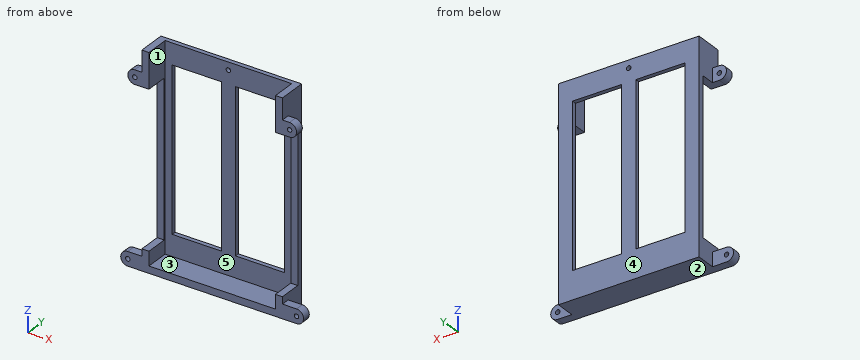
```python
from build123d import *

# Parameters (mm, degrees)
SKETCH_2_W          = 100
SKETCH_2_H          = 40
EXTRUDE_1_DEPTH     = 150
SKETCH_3_W          = 90
SKETCH_3_H          = 32
CUT_EXTRUDE_1_DEPTH = 145
SKETCH_4_W          = 30
SKETCH_4_H          = 115
CUT_EXTRUDE_2_DEPTH = 20
SKETCH_5_W          = 35
SKETCH_5_H          = 115
CUT_EXTRUDE_3_DEPTH = 20
SKETCH_6_W          = 120
SKETCH_6_H          = 31
CUT_EXTRUDE_4_DEPTH = 207
SKETCH_7_R          = 1.5
CUT_EXTRUDE_5_DEPTH = 15
SKETCH_8_R          = 2.5
CUT_EXTRUDE_6_DEPTH = 15
SKETCH_10_W         = 4
SKETCH_10_H         = 18
EXTRUDE_2_DEPTH     = 5
SKETCH_11_W         = 100
SKETCH_11_H         = 150
CUT_EXTRUDE_7_DEPTH = 20
SKETCH_12_R         = 1.6
EXTRUDE_5_DEPTH     = 6
EXTRUDE_6_REACH     = 166.076
SKETCH_13_W         = 4.955411511
SKETCH_13_H         = 10
SKETCH_13_W_2       = 5.044588489
SKETCH_14_R         = 1.6
CUT_EXTRUDE_8_DEPTH = 10


with BuildPart() as part:
    # 草图2 → 凸台-拉伸1 (new body)
    with BuildSketch(Plane.XY):
        Rectangle(SKETCH_2_W, SKETCH_2_H)
    extrude(amount=EXTRUDE_1_DEPTH)

    # 草图3 → 切除-拉伸1 (cut)
    with BuildSketch(Plane.XY.offset(150)):
        with Locations((0.044588489, 1)):
            Rectangle(SKETCH_3_W, SKETCH_3_H)
    extrude(amount=-CUT_EXTRUDE_1_DEPTH, mode=Mode.SUBTRACT)

    # 草图4 → 切除-拉伸2 (cut)
    with BuildSketch(Plane.XZ.offset(20)):
        with Locations((-25, 77.5)):
            Rectangle(SKETCH_4_W, SKETCH_4_H)
        with Locations((25, 77.5)):
            Rectangle(SKETCH_4_W, SKETCH_4_H)
    extrude(amount=-CUT_EXTRUDE_2_DEPTH, mode=Mode.SUBTRACT)

    # 草图5 → 切除-拉伸3 (cut)
    with BuildSketch(Plane(origin=(0, 20, 0), x_dir=(1, 0, 0), z_dir=(0, 1, 0))):
        with Locations((-22.5, -77.5)):
            Rectangle(SKETCH_5_W, SKETCH_5_H)
        with Locations((22.5, -77.5)):
            Rectangle(SKETCH_5_W, SKETCH_5_H)
    extrude(amount=-CUT_EXTRUDE_3_DEPTH, mode=Mode.SUBTRACT)

    # 草图6 → 切除-拉伸4 (cut)
    with BuildSketch(Plane.ZY.offset(50)):
        with Locations((75, 0.5)):
            Rectangle(SKETCH_6_W, SKETCH_6_H)
    extrude(amount=-CUT_EXTRUDE_4_DEPTH, mode=Mode.SUBTRACT)

    # 草图7 → 切除-拉伸5 (cut)
    with BuildSketch(Plane.XZ.offset(20)):
        with Locations(Location((-5, 134, 0), (0, 0, 270))):
            Circle(SKETCH_7_R)
        with Locations(Location((5, 134, 0), (0, 0, 270))):
            Circle(SKETCH_7_R)
        with Locations(Location((5, 124, 0), (0, 0, 270))):
            Circle(SKETCH_7_R)
        with Locations(Location((-5, 124, 0), (0, 0, 270))):
            Circle(SKETCH_7_R)
    extrude(amount=-CUT_EXTRUDE_5_DEPTH, mode=Mode.SUBTRACT)

    # 草图8 → 切除-拉伸6 (cut)
    with BuildSketch(Plane.XZ.offset(20)):
        with Locations(Location((0, 129, 0), (0, 0, 270))):
            Circle(SKETCH_8_R)
    extrude(amount=-CUT_EXTRUDE_6_DEPTH, mode=Mode.SUBTRACT)

    # 草图10 → 凸台-拉伸2 (add)
    with BuildSketch(Plane.XZ.offset(20)):
        with Locations((-12, 126)):
            Rectangle(SKETCH_10_W, SKETCH_10_H)
        with Locations((12, 126)):
            Rectangle(SKETCH_10_W, SKETCH_10_H)
    extrude(amount=-EXTRUDE_2_DEPTH)

    # 草图11 → 切除-拉伸7 (cut)
    with BuildSketch(Plane.XZ.offset(20)):
        with Locations((0, 75)):
            Rectangle(SKETCH_11_W, SKETCH_11_H)
    extrude(amount=-CUT_EXTRUDE_7_DEPTH, mode=Mode.SUBTRACT)

    # 草图12 → 凸台-拉伸5 (add)
    # profile 1 of 4: a face of its own
    with BuildSketch(Plane.XZ):
        with BuildLine():
            Line((-44.955411511, 135), (-54.955411511, 135))
            ThreePointArc((-54.955411511, 135), (-59.955411511, 130), (-54.955411511, 125))
            Line((-54.955411511, 125), (-44.955411511, 125))
            Line((-44.955411511, 125), (-44.955411511, 135))
        make_face()
        with Locations(Location((-54.955411511, 130, 0), (0, 0, 270))):
            Circle(SKETCH_12_R, mode=Mode.SUBTRACT)
    # profile 2 of 4: a face of its own
    with BuildSketch(Plane.XZ):
        with BuildLine():
            Line((50, 0), (60, 0))
            ThreePointArc((60, 0), (65, 5), (60, 10))
            Line((60, 10), (50, 10))
            Line((50, 10), (50, 0))
        make_face()
        with Locations(Location((60, 5, 0), (0, 0, 270))):
            Circle(SKETCH_12_R, mode=Mode.SUBTRACT)
    # profile 3 of 4: a face of its own
    with BuildSketch(Plane.XZ):
        with BuildLine():
            Line((45.044588489, 135), (55.044588489, 135))
            ThreePointArc((55.044588489, 135), (60.044588489, 130), (55.044588489, 125))
            Line((55.044588489, 125), (45.044588489, 125))
            Line((45.044588489, 125), (45.044588489, 135))
        make_face()
        with Locations(Location((55.044588489, 130, 0), (0, 0, 270))):
            Circle(SKETCH_12_R, mode=Mode.SUBTRACT)
    # profile 4 of 4: a face of its own
    with BuildSketch(Plane.XZ):
        with BuildLine():
            Line((-50, 0), (-60, 0))
            ThreePointArc((-60, 0), (-65, 5), (-60, 10))
            Line((-60, 10), (-50, 10))
            Line((-50, 10), (-50, 0))
        make_face()
        with Locations(Location((-60, 5, 0), (0, 0, 270))):
            Circle(SKETCH_12_R, mode=Mode.SUBTRACT)
    extrude(amount=-EXTRUDE_5_DEPTH)

    # 草图13 → 凸台-拉伸6 (add, up to next)
    with BuildSketch(Plane(origin=(0, 6, 0), x_dir=(1, 0, 0), z_dir=(0, 1, 0)), mode=Mode.PRIVATE) as extrude_6_sk1:
        with Locations((47.522294245, -130)):
            Rectangle(SKETCH_13_W, SKETCH_13_H)
    extrude_6_tool1 = extrude(extrude_6_sk1.sketch, amount=EXTRUDE_6_REACH, mode=Mode.PRIVATE) - part.part
    # 草图13 → 凸台-拉伸6 (add, up to next)
    with BuildSketch(Plane(origin=(0, 6, 0), x_dir=(1, 0, 0), z_dir=(0, 1, 0)), mode=Mode.PRIVATE) as extrude_6_sk2:
        with Locations((-47.477705755, -130)):
            Rectangle(SKETCH_13_W_2, SKETCH_13_H)
    extrude_6_tool2 = extrude(extrude_6_sk2.sketch, amount=EXTRUDE_6_REACH, mode=Mode.PRIVATE) - part.part
    add(extrude_6_tool1.solids().sort_by_distance((47.522294, 6, 130))[0])
    add(extrude_6_tool2.solids().sort_by_distance((-47.477706, 6, 130))[0])

    # 草图14 → 切除-拉伸8 (cut)
    with BuildSketch(Plane(origin=(0, 20, 0), x_dir=(1, 0, 0), z_dir=(0, 1, 0))):
        with Locations(Location((0, -144.5, 0), (0, 0, 270))):
            Circle(SKETCH_14_R)
    extrude(amount=-CUT_EXTRUDE_8_DEPTH, mode=Mode.SUBTRACT)


solid = part.part
```
Check sheet for the modelled part. Datum: model origin and axes. Units: mm. Face numbers are marked on the shaded views. A direction names the side the tool comes from. Round coordinates to 2 decimals unless told otherwise and drop trailing zeros. Order: outer loops, then holes, each group sorted by start corner. A loop starts at its lowest first (then second) coordinate and runs counter-clockwise, first axis right, second up. Notation, with made-up numbers: M 87,24.5 L 100,24.5 A14 cw 100,40.5 Z; hole C -23,-32 d4. An arc over 180 degrees is marked long. Answer in a Markdown table with one row per item.
(1) Gauge pin test, flat ends, axial feed: pin 1 (3 mm diameter, centred on y = 17.5, z = 19, fed in from +X); pin 2 (3.5 mm diameter, centred on y = 18.5, z = 76.5, fed in from -X); pin 3 (1.8 mm diameter, centred on x = 57.5, y = 4.5, fed in from +Z). Record the tip position at first contact, or that the pin passes through.
Findings:
| item | result |
|---|---|
| pin 1 | stops at x = 50 |
| pin 2 | stops at x = -50 |
| pin 3 | stops at z = 134.75 |
(2) Set-up check for the marked faces 4 and 5: record each of +Z, -Z, +X, -X, +Y, -Y from which the full face is reachable in a straight line by a thin tool's end or side.
Findings:
| item | result |
|---|---|
| face 4 | +Z, -Z, +X, -X, +Y |
| face 5 | +Z, -Y |
(3) Section check D-D on z = 51.5. Record the boundary of the cut face in (x, y), plus the area to 3 significant figures.
Findings:
| item | result |
|---|---|
| outline | M -50,16 L -44.96,16 L -44.96,17 L -40,17 L -40,20 L -50,20 Z; M -5,17 L 5,17 L 5,20 L -5,20 Z; M 40,17 L 45.04,17 L 45.04,16 L 50,16 L 50,20 L 40,20 Z |
| area | 100 mm^2 |
(4) Material ranges on line 1 along X through (y, z) = (4.7, 130); line 2 along X through (y, z) = (10.25, 138); line 3 along Z through (x, y) = (55.5, 3.25), recorded low to high. Write a range as from..to.
Findings:
| item | result |
|---|---|
| line 1 | x = -59.96..-56.56, -53.36..-44.96, 45.04..53.44, 56.64..60.04 |
| line 2 | x = -50..-44.96, 45.04..50 |
| line 3 | z = 0..10, 125.02..128.47, 131.53..134.98 |
(5) Draft check along X on the marked faces 1, 2 and 3. Enter one of: +X half, -X half, draft (parallel to the pull), parting line (faces both ways), or undercut.
Findings:
| item | result |
|---|---|
| face 1 | undercut |
| face 2 | draft |
| face 3 | undercut |
(6) Section check B-B on z = 144.5. Record the boundary of the cut face in (x, y), plus the area to 3 significant figures.
Findings:
| item | result |
|---|---|
| outline | M -50,0 L -44.96,0 L -44.96,17 L -1.6,17 L -1.6,20 L -50,20 Z; M 1.6,17 L 45.04,17 L 45.04,0 L 50,0 L 50,20 L 1.6,20 Z |
| area | 460 mm^2 |
(7) Section check C-C on x = 0. Record the boundary of the cut face in (y, z), plus the area to 3 significant figures.
Findings:
| item | result |
|---|---|
| outline | M 0,0 L 20,0 L 20,142.9 L 17,142.9 L 17,5 L 0,5 Z; M 17,146.1 L 20,146.1 L 20,150 L 17,150 Z |
| area | 525 mm^2 |
(8) Section check A-A on y = 1.75. Record the boundary of the cut face in (x, z).
Findings:
| item | result |
|---|---|
| outline | M -60,0 L 60,0 A5 ccw 60,10 L 50,10 L 50,15 L 45.04,15 L 45.04,5 L -44.96,5 L -44.96,15 L -50,15 L -50,10 L -60,10 A5 ccw Z; M -54.96,125 L -44.96,125 L -44.96,150 L -50,150 L -50,135 L -54.96,135 A5 ccw Z; M 45.04,125 L 55.04,125 A5 ccw 55.04,135 L 50,135 L 50,150 L 45.04,150 Z; hole C -60,5 d3.2; hole C -54.96,130 d3.2; hole C 55.04,130 d3.2; hole C 60,5 d3.2 |
